Input: dimensioned drawing with shaded views. Units: mm. Origin: part minimum x, y, z. A direction names the side the tool comes from. Give positions to 0.01 mm unless a question says otherwise; leave off trailing zeros. Order: outer loops, then holes, each group sorted by start corner. A loop starts at its lowest first (then second) coordinate and runs counter-clockwise, first axis right, second up.
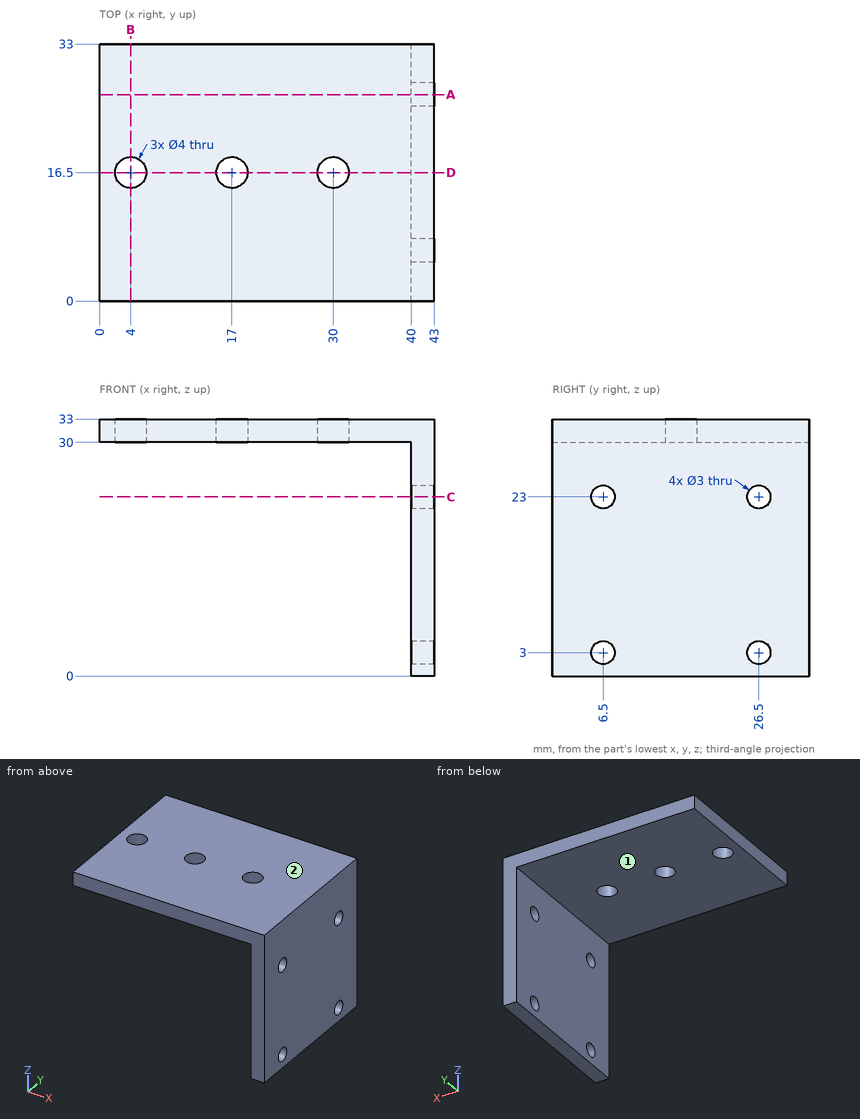
1) Section query A-A, the plane y = 26.5. Return the cut outline in (x, z).
Report:
outline: (0, 30) - (40, 30) - (40, 24.5) - (43, 24.5) - (43, 33) - (0, 33) - close; (40, 0) - (43, 0) - (43, 1.5) - (40, 1.5) - close; (40, 4.5) - (43, 4.5) - (43, 21.5) - (40, 21.5) - close
2) Section query C-C, the plane z = 23. Return the cut outline in (x, y).
Report:
outline: (40, 0) - (43, 0) - (43, 5) - (40, 5) - close; (40, 8) - (43, 8) - (43, 25) - (40, 25) - close; (40, 28) - (43, 28) - (43, 33) - (40, 33) - close
3) Section query D-D, the plane y = 16.5. Return the cut outline in (x, z).
Report:
outline: (0, 30) - (2, 30) - (2, 33) - (0, 33) - close; (6, 30) - (15, 30) - (15, 33) - (6, 33) - close; (19, 30) - (28, 30) - (28, 33) - (19, 33) - close; (32, 30) - (40, 30) - (40, 0) - (43, 0) - (43, 33) - (32, 33) - close
4) Section query B-B, the plane x = 4. Return the cut outline in (y, z).
Report:
outline: (0, 30) - (14.5, 30) - (14.5, 33) - (0, 33) - close; (18.5, 30) - (33, 30) - (33, 33) - (18.5, 33) - close
5) Reachability of the marked faces 1 and 2 from +Z, -Z, +X, -X, +Y, -Y: full face, straight path, thin tool, end or side. Return the list, or none.
Report:
face 1: -Z, -X, +Y, -Y
face 2: +Z, +X, -X, +Y, -Y
6) Pin query (flat end, axial travel): pin 1 (3.5 mm diameter, centred on y = 6.5, z = 23, fed in from -X); pin 2 (4.5 mm diameter, centred on x = 4, y = 16.5, fed in from +Z); pin 3 (10 mm diameter, centred on x = 19, y = 19, fed in from -Z). Return the tip coordinate at first contact, or that it passes through.
Report:
pin 1: stops at x = 40
pin 2: stops at z = 33
pin 3: stops at z = 30
7) Material intervals for L1, parallel to Y at x = 41.8, z = 3; L2, parallel to X at y = 23.5, z = 4; L3, parallel to X at y = 16, z = 31, sorted ascending.
Report:
L1: y = 0 to 5, 8 to 25, 28 to 33
L2: x = 40 to 43
L3: x = 0 to 2.06, 5.94 to 15.06, 18.94 to 28.06, 31.94 to 43
